Design review of the part built by this model. Coordinates are the model's own, in mm. Face numbers are marked on the shaded views. Coordinates: 2 decimals unless noted, no trailing zeros. Loops run counter-clockwise (first coordinate to the right, second up) from the corner with the lowest first, then second, coordinate; pieces in that order, holes last. Notation, with made-up numbers: (29.25, 44) - (71.25, 44) arc R15 cw to (71.25, 62) - close; hole circle Ø2 at (-39.5, 12). An arc over 180 degrees is marked (long way). Use one line per item in the form item = value. Start each with the question number.
(1) Clearance check with flat-ended pins moving along their axes: pin 1 Ø5 at (x, z) = (49.23, 28.51) entering from +Y; pin 2 Ø4 at (x, z) = (-45, 87) entering from +Y; pin 3 Ø1.5 at (y, z) = (3.5, 129) entering from -X; pin 4 Ø2 at (x, y) = (45, 1.5) entering from -Z. State where each tip first meets the part, or that it passes through.
(2) Add section A-A (x = -24). State the section outline as (y, z) points, plus the area to 3 significant figures.
(3) The part is to be moulded in two halves that separate along X. For the marked faces 1 and 2, say which applies: pulls with the +X half, pulls with the -X half, needs draft (parallel to the pull), parting line crosses it, or undercut.
(4) Add section B-B (z = 101.5). State the section outline as (x, y) points, plus the area to 3 significant figures.
(5) For L1, parallel to X at y = 3.4, z = 97; L2, parallel to Z at x = 28, y = 2.95; L3, parallel to X at y = 3.85, z = 30.5, list the stretches that pass through material, from the lowest coordinate up.
(6) Add section C-C (y = 0.85). Count the separate pieces of the cut face and the enclosed holes in it, plus the area to 3 significant figures.
```python
from build123d import *

# Parameters (mm, degrees)
SKETCH1_W           = 133.2946
SKETCH1_H           = 90.45
BOSS_EXTRUDE1_DEPTH = 5
SKETCH2_W           = 10
SKETCH2_H           = 10
BOSS_EXTRUDE2_DEPTH = 5
SKETCH4_R           = 3.25
CUT_EXTRUDE1_DEPTH  = 5
FILLET1_R           = 2.5
CUT_EXTRUDE2_DEPTH  = 3
FILLET2_R           = 1
FILLET3_R           = 0.5


with BuildPart() as part:
    # Sketch1 → Boss-Extrude1 (new body)
    with BuildSketch(Plane(origin=(0, 0, 0), x_dir=(1, 0, 0), z_dir=(0, 1, 0))):
        with Locations((-2.415435148, -78.733798602)):
            Rectangle(SKETCH1_W, SKETCH1_H)
    extrude(amount=BOSS_EXTRUDE1_DEPTH)

    # Sketch2 → Boss-Extrude2 (add)
    with BuildSketch(Plane(origin=(0, 5, 0), x_dir=(1, 0, 0), z_dir=(0, 1, 0))):
        with Locations((-54.062735148, -28.508798602)):
            Rectangle(SKETCH2_W, SKETCH2_H)
        with Locations((49.231864852, -28.508798602)):
            Rectangle(SKETCH2_W, SKETCH2_H)
        with Locations((49.231864852, -128.958798602)):
            Rectangle(SKETCH2_W, SKETCH2_H)
        with Locations((-54.062735148, -128.958798602)):
            Rectangle(SKETCH2_W, SKETCH2_H)
    extrude(amount=-BOSS_EXTRUDE2_DEPTH)

    # Sketch4 → Cut-Extrude1 (cut)
    with BuildSketch(Plane(origin=(0, 5, 0), x_dir=(1, 0, 0), z_dir=(0, 1, 0))):
        with Locations(Location((49.231864852, -28.508798602, 0), (0, 0, 270))):
            Circle(SKETCH4_R)
        with Locations(Location((-54.062735148, -28.508798602, 0), (0, 0, 270))):
            Circle(SKETCH4_R)
        with Locations(Location((-54.062735148, -128.958798602, 0), (0, 0, 270))):
            Circle(SKETCH4_R)
        with Locations(Location((49.231864852, -128.958798602, 0), (0, 0, 270))):
            Circle(SKETCH4_R)
    extrude(amount=-CUT_EXTRUDE1_DEPTH, mode=Mode.SUBTRACT)

    # Fillet1
    fillet1_edges = [part.edges().sort_by_distance(p)[0] for p in [
        (-59.062735148, 2.5, 33.508798602),
        (-59.062735148, 2.5, 23.508798602),
        (-49.062735148, 2.5, 23.508798602),
        (-49.062735148, 2.5, 33.508798602),
        (44.231864852, 2.5, 33.508798602),
        (44.231864852, 2.5, 23.508798602),
        (54.231864852, 2.5, 23.508798602),
        (54.231864852, 2.5, 33.508798602),
        (54.231864852, 2.5, 123.958798602),
        (54.231864852, 2.5, 133.958798602),
        (44.231864852, 2.5, 133.958798602),
        (44.231864852, 2.5, 123.958798602),
        (-49.062735148, 2.5, 123.958798602),
        (-49.062735148, 2.5, 133.958798602),
        (-59.062735148, 2.5, 133.958798602),
        (-59.062735148, 2.5, 123.958798602),
    ]]
    fillet(fillet1_edges, radius=FILLET1_R)

    # Sketch6 → Cut-Extrude2 (cut)
    with BuildSketch(Plane(origin=(0, 5, 0), x_dir=(1, 0, 0), z_dir=(0, 1, 0))):
        Polygon((-58.965485148, -119.958798602), (60.166814852, -119.958798602), (60.166814852, -37.508798602), (-58.965485148, -37.508798602), (-64.997685148, -43.148798602), (-64.997685148, -114.318798602), align=None)
    extrude(amount=-CUT_EXTRUDE2_DEPTH, mode=Mode.SUBTRACT)

    # Fillet2
    fillet2_edges = [part.edges().sort_by_distance(p)[0] for p in [
        (60.166814852, 3.5, 37.508798602),
        (60.166814852, 3.5, 119.958798602),
    ]]
    fillet(fillet2_edges, radius=FILLET2_R)

    # Fillet3
    fillet3_edges = [part.edges().sort_by_distance(p)[0] for p in [
        (-58.965485148, 3.5, 37.508798602),
        (-58.965485148, 3.5, 119.958798602),
        (-64.997685148, 3.5, 114.318798602),
        (-64.997685148, 3.5, 43.148798602),
    ]]
    fillet(fillet3_edges, radius=FILLET3_R)


solid = part.part
```
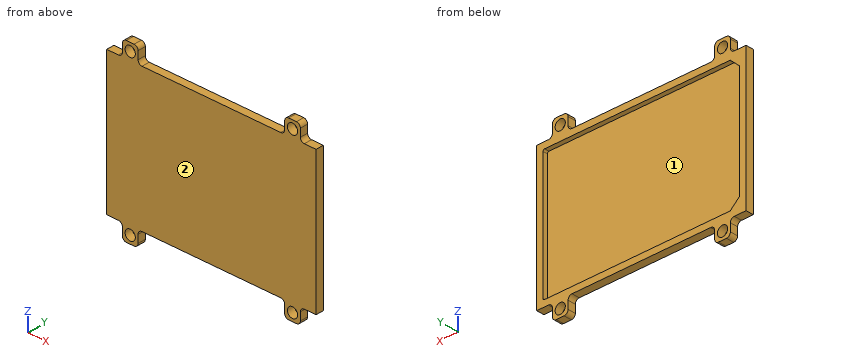
Computed values:
q1.pin_1 = through
q1.pin_2 = 2
q1.pin_3 = -59.06
q1.pin_4 = 23.62
q2.outline = (0, 33.51) - (5, 33.51) - (5, 37.51) - (2, 37.51) - (2, 119.96) - (5, 119.96) - (5, 123.96) - (0, 123.96) - close
q2.area = 205 mm^2
q3.face_1 = undercut
q3.face_2 = needs draft
q4.outline = (-69.06, 0) - (64.23, 0) - (64.23, 5) - (60.17, 5) - (60.17, 2) - (-65, 2) - (-65, 5) - (-69.06, 5) - close
q4.area = 291 mm^2
q5.L1 = -69.06 to -65, 60.17 to 64.23
q5.L2 = 33.51 to 37.51, 119.96 to 123.96
q5.L3 = -59.06 to -56.63, -51.49 to -49.06, 44.23 to 46.66, 51.8 to 54.23
q6.separate_pieces = 1
q6.enclosed_holes = 4
q6.area = 12,300 mm^2
